```python
from build123d import *

# Parameters (mm, degrees)
SKETCH1_R                = 12.7
BOSS_EXTRUDE1_DEPTH      = 4.7752
SKETCH2_R                = 7.1501
BOSS_EXTRUDE2_DEPTH      = 24.13
SKETCH3_R                = 1.8288
BOSS_EXTRUDE3_DEPTH      = 12.7
BOSS_EXTRUDE3_DEPTH_BACK = 17.78


with BuildPart() as part:
    # Sketch1 → Boss-Extrude1 (new body)
    with BuildSketch(Plane.XY):
        Circle(SKETCH1_R)
    extrude(amount=BOSS_EXTRUDE1_DEPTH)

    # Sketch2 → Boss-Extrude2 (add)
    with BuildSketch(Plane(origin=(0, 0, 0), x_dir=(-1, 0, 0), z_dir=(0, 0, -1))):
        Circle(SKETCH2_R)
    extrude(amount=BOSS_EXTRUDE2_DEPTH)

    # Sketch3 → Boss-Extrude3 (add, two sides)
    with BuildSketch(Plane.XY.offset(4.7752)) as boss_extrude3_sk:
        with Locations((0, 9.525)):
            Circle(SKETCH3_R)
        with Locations((8.248891971, 4.7625)):
            Circle(SKETCH3_R)
        with Locations((8.248891971, -4.7625)):
            Circle(SKETCH3_R)
        with Locations((0, -9.525)):
            Circle(SKETCH3_R)
        with Locations((-8.248891971, -4.7625)):
            Circle(SKETCH3_R)
        with Locations((-8.248891971, 4.7625)):
            Circle(SKETCH3_R)
    extrude(amount=BOSS_EXTRUDE3_DEPTH)
    extrude(boss_extrude3_sk.sketch, amount=-BOSS_EXTRUDE3_DEPTH_BACK)


solid = part.part
```
Build history of the part. All positions in model axes, mm. A direction names the side the tool comes from. Round coordinates to 2 decimals unless told otherwise and drop trailing zeros. Order: outer loops, then holes, each group sorted by start corner. A loop starts at its lowest first (then second) coordinate and runs counter-clockwise, first axis right, second up. Notation, with made-up numbers: (-11.5, 57.25) - (17.5, 57.25) arc R14 cw to (17.5, 72.25) - close; hole circle Ø7 at (66, 58.25). An arc over 180 degrees is marked (long way). Use a Markdown table: item, result.
1) Tool access for faces 5 (the face through (-0.4, 7.74, -6.41)), 6 (the face through (0, 10, -13.005)), 7 (the face through (0, -9, -13.005)): list every direction of +Z, -Z, +X, -X, +Y, -Y with a clear straight run to the whole face (end or side of a thin tool).
Recorded:
| item | result |
|---|---|
| face 5 | -Z |
| face 6 | -Z, +X, -X, +Y |
| face 7 | -Z, +X, -X, -Y |
2) Flat gauge pins, fed straight in: pin 1 Ø10 at (x, z) = (6.5, -15.5) entering from +Y; pin 2 Ø3 at (x, y) = (-9, -4) entering from -Z; pin 3 Ø1 at (x, z) = (-9.5, -2.5) entering from -Y; pin 4 Ø12.5 at (x, y) = (2, 3) entering from +Z. Where does each tip first touch, or does it go through?
Recorded:
| item | result |
|---|---|
| pin 1 | stops at y = 6.99 |
| pin 2 | stops at z = -13 |
| pin 3 | stops at y = -6.43 |
| pin 4 | stops at z = 17.48 |
3) Pull direction Y, two halves, no side cores. Call faces 1 (the face through (-0.24, -7.71, -6.41)), 2 (the face through (-9.597, 5.998, 11.036)), 3 (the face through (-2.75, -12.4, 2.35)), 4 (the face through (8, -5, 17.475)): pulls with the +Y half, pulls with the -Y half, needs draft (parallel to the pull), parting line crosses it, or undercut.
Recorded:
| item | result |
|---|---|
| face 1 | undercut |
| face 2 | undercut |
| face 3 | parting line crosses it |
| face 4 | needs draft |
4) Saw through at D-D on z = -21. Write the cut outline in (x, y).
Recorded:
| item | result |
|---|---|
| outline | circle Ø14.3 at (0, 0) |
5) Saw through at C-C on x = 0. Write the cut outline in (y, z).
Recorded:
| item | result |
|---|---|
| outline | (-12.7, 0) - (-11.35, 0) - (-11.35, -13) - (-7.7, -13) - (-7.7, 0) - (-7.15, 0) - (-7.15, -24.13) - (7.15, -24.13) - (7.15, 0) - (7.7, 0) - (7.7, -13) - (11.35, -13) - (11.35, 0) - (12.7, 0) - (12.7, 4.78) - (11.35, 4.78) - (11.35, 17.48) - (7.7, 17.48) - (7.7, 4.78) - (-7.7, 4.78) - (-7.7, 17.48) - (-11.35, 17.48) - (-11.35, 4.78) - (-12.7, 4.78) - close |
6) Saw through at B-B on y = 0. Write the cut outline in (x, z), and give its area (3 significant figures).
Recorded:
| item | result |
|---|---|
| outline | (-12.7, 0) - (-7.15, 0) - (-7.15, -24.13) - (7.15, -24.13) - (7.15, 0) - (12.7, 0) - (12.7, 4.78) - (-12.7, 4.78) - close |
| area | 466 mm² |
7) Saw through at A-A on z = -8. Write the cut outline in (x, y) (1 decimal).
Recorded:
| item | result |
|---|---|
| outline | circle Ø3.7 at (-8.2, -4.8); circle Ø3.7 at (-8.2, 4.8); circle Ø14.3 at (0, 0); circle Ø3.7 at (0, -9.5); circle Ø3.7 at (0, 9.5); circle Ø3.7 at (8.2, -4.8); circle Ø3.7 at (8.2, 4.8) |
8) Wall check: L1, parallel to X at y = 4.75, z = 9.5; L2, parallel to X at y = 4.5, z = -4; L3, parallel to Y at x = -8.25, z = 13. Give the ranges that are in metal, low to high.
Recorded:
| item | result |
|---|---|
| L1 | x = -10.08 to -6.42, 6.42 to 10.08 |
| L2 | x = -10.06 to -6.44, -5.56 to 5.56, 6.44 to 10.06 |
| L3 | y = -6.59 to -2.93, 2.93 to 6.59 |
